```python
from build123d import *

# Parameters (mm, degrees)
PAD001_DEPTH      = 5
THICKNESS001_T    = 1.5
BOX_W             = 2
BOX_H             = 8
BOX_DEPTH         = 5
BOX001_W          = 2
BOX001_H          = 8
BOX001_DEPTH      = 5
BOX002_W          = 2
BOX002_H          = 6
BOX002_DEPTH      = 5
BOX003_W          = 2
BOX003_H          = 6
BOX003_DEPTH      = 5
CYLINDER001_W     = 3
CYLINDER001_H     = 5
CYLINDER001_ANGLE = 180
BOX005_W          = 6
BOX005_H          = 0.6
BOX005_DEPTH      = 5
CYLINDER005_W     = 3
CYLINDER005_H     = 5
CYLINDER005_ANGLE = 180
BOX007_W          = 6
BOX007_H          = 0.6
BOX007_DEPTH      = 5
SKETCH002_R       = 2.65
SKETCH002_R_2     = 1.25
SKETCH002_R_3     = 1
SKETCH002_W       = 5.3
SKETCH002_H       = 10.4
POCKET_DEPTH      = 6.501
BOX008_W          = 8
BOX008_H          = 2
BOX008_DEPTH      = 4.9
BOX009_W          = 8
BOX009_H          = 2
BOX009_DEPTH      = 4.9
SKETCH006_R       = 2.65
PAD003_DEPTH      = 3.5
SKETCH007_R       = 1.35
POCKET002_DEPTH   = 3.5


with BuildPart() as part:
    # Sketch001 → Pad001 (new body)
    with BuildSketch(Plane.XY):
        with BuildLine():
            Line((2, 31.1), (55.5, 31.1))
            ThreePointArc((57.6, 29), (56.984924, 30.484924), (55.5, 31.1))
            Line((57.6, 29), (57.6, 2))
            ThreePointArc((55.5, -0.1), (56.984924, 0.515076), (57.6, 2))
            Line((55.5, -0.1), (2, -0.1))
            ThreePointArc((-0.1, 2), (0.515076, 0.515076), (2, -0.1))
            Line((-0.1, 2), (-0.1, 29))
            ThreePointArc((2, 31.1), (0.515076, 30.484924), (-0.1, 29))
        make_face()
    extrude(amount=PAD001_DEPTH)

    # Thickness001
    thickness001_openings = [part.faces().sort_by_distance(p)[0] for p in [
        (28.75, 15.5, 0),
    ]]
    offset(amount=THICKNESS001_T, openings=thickness001_openings)

    # Box → Box (cut)
    with BuildSketch(Plane(origin=(57.5, 1.5, 0), x_dir=(1, 0, 0), z_dir=(0, 0, 1))):
        with Locations((1, 4)):
            Rectangle(BOX_W, BOX_H)
    extrude(amount=BOX_DEPTH, mode=Mode.SUBTRACT)

    # Box001 → Box001 (cut)
    with BuildSketch(Plane(origin=(57.5, 11.08, 0), x_dir=(1, 0, 0), z_dir=(0, 0, 1))):
        with Locations((1, 4)):
            Rectangle(BOX001_W, BOX001_H)
    extrude(amount=BOX001_DEPTH, mode=Mode.SUBTRACT)

    # Box002 → Box002 (cut)
    with BuildSketch(Plane(origin=(57.5, 20.575, 0), x_dir=(1, 0, 0), z_dir=(0, 0, 1))):
        with Locations((1, 3)):
            Rectangle(BOX002_W, BOX002_H)
    extrude(amount=BOX002_DEPTH, mode=Mode.SUBTRACT)

    # Box003 → Box003 (cut)
    with BuildSketch(Plane(origin=(-2, 10.35, 0), x_dir=(1, 0, 0), z_dir=(0, 0, 1))):
        with Locations((1, 3)):
            Rectangle(BOX003_W, BOX003_H)
    extrude(amount=BOX003_DEPTH, mode=Mode.SUBTRACT)

    # Cylinder001 → Cylinder001 (revolve)
    with BuildSketch(Plane(origin=(16, 0.5, 0), x_dir=(1, 0, 0), z_dir=(0, -1, 0))):
        with Locations((1.5, 2.5)):
            Rectangle(CYLINDER001_W, CYLINDER001_H)
    revolve(axis=Axis((16, 0.5, 0), (0, 0, 1)), revolution_arc=CYLINDER001_ANGLE)

    # Box005 → Box005 (join)
    with BuildSketch(Plane(origin=(13, -0.1, 0), x_dir=(1, 0, 0), z_dir=(0, 0, 1))):
        with Locations((3, 0.3)):
            Rectangle(BOX005_W, BOX005_H)
    extrude(amount=BOX005_DEPTH)

    # Cylinder005 → Cylinder005 (revolve)
    with BuildSketch(Plane(origin=(42.25, 30.5, 0), x_dir=(-1, 0, 0), z_dir=(0, 1, 0))):
        with Locations((1.5, 2.5)):
            Rectangle(CYLINDER005_W, CYLINDER005_H)
    revolve(axis=Axis((42.25, 30.5, 0), (0, 0, 1)), revolution_arc=CYLINDER005_ANGLE)

    # Box007 → Box007 (join)
    with BuildSketch(Plane(origin=(39.25, 30.5, 0), x_dir=(1, 0, 0), z_dir=(0, 0, 1))):
        with Locations((3, 0.3)):
            Rectangle(BOX007_W, BOX007_H)
    extrude(amount=BOX007_DEPTH)

    # Sketch002 → Pocket (cut, through all)
    with BuildSketch(Plane.XY):
        with Locations((47.135, 17.52)):
            Circle(SKETCH002_R)
        with Locations((16, 0.5)):
            Circle(SKETCH002_R_2)
        with Locations((42.25, 30.5)):
            Circle(SKETCH002_R_2)
        with Locations((45.15, 2.85)):
            Circle(SKETCH002_R_3)
        with Locations((33.1, 27.275)):
            Circle(SKETCH002_R_3)
        with Locations((3.6, 25.39)):
            Rectangle(SKETCH002_W, SKETCH002_H)
        with Locations((47.2, 25.7)):
            Rectangle(SKETCH002_W, SKETCH002_H)
        with BuildLine():
            Line((30.2, 2.925), (37, 2.925))
            ThreePointArc((37, 2.925), (37.919239, 3.305761), (38.3, 4.225))
            Line((38.3, 5.125), (38.3, 4.225))
            ThreePointArc((38.3, 5.125), (37.919239, 6.044239), (37, 6.425))
            Line((37, 6.425), (30.2, 6.425))
            ThreePointArc((30.2, 6.425), (29.280761, 6.044239), (28.9, 5.125))
            Line((28.9, 5.125), (28.9, 4.225))
            ThreePointArc((28.9, 4.225), (29.280761, 3.305761), (30.2, 2.925))
        make_face()
    extrude(amount=POCKET_DEPTH, mode=Mode.SUBTRACT)

    # Cone → Cone (revolve, cut)
    with BuildSketch(Plane(origin=(16, 0.5, 5.8), x_dir=(1, 0, 0), z_dir=(0, -1, 0))):
        Polygon((0, 0), (1.15, 0), (1.75, 0.7), (0, 0.7), align=None)
    revolve(axis=Axis((16, 0.5, 5.8), (0, 0, 1)), mode=Mode.SUBTRACT)

    # Cone001 → Cone001 (revolve, cut)
    with BuildSketch(Plane(origin=(42.25, 30.5, 5.8), x_dir=(1, 0, 0), z_dir=(0, -1, 0))):
        Polygon((0, 0), (1.15, 0), (1.75, 0.7), (0, 0.7), align=None)
    revolve(axis=Axis((42.25, 30.5, 5.8), (0, 0, 1)), mode=Mode.SUBTRACT)

    # Box008 → Box008 (cut)
    with BuildSketch(Plane(origin=(10.35, 31, 0), x_dir=(1, 0, 0), z_dir=(0, 0, 1))):
        with Locations((4, 1)):
            Rectangle(BOX008_W, BOX008_H)
    extrude(amount=BOX008_DEPTH, mode=Mode.SUBTRACT)

    # Box009 → Box009 (cut)
    with BuildSketch(Plane(origin=(21.82, 31, 0), x_dir=(1, 0, 0), z_dir=(0, 0, 1))):
        with Locations((4, 1)):
            Rectangle(BOX009_W, BOX009_H)
    extrude(amount=BOX009_DEPTH, mode=Mode.SUBTRACT)

    # Sketch006 → Pad003 (join)
    with BuildSketch(Plane.XY.offset(5)):
        with Locations((14.8, 22.4)):
            Circle(SKETCH006_R)
        with Locations((49.8, 5.4)):
            Circle(SKETCH006_R)
        with Locations((40.8, 22.4)):
            Circle(SKETCH006_R)
        with Locations((14.8, 5.4)):
            Circle(SKETCH006_R)
    extrude(amount=-PAD003_DEPTH)

    # Sketch007 → Pocket002 (cut)
    with BuildSketch(Plane.XY.offset(6.5)):
        with Locations((14.8, 22.4)):
            Circle(SKETCH007_R)
        with Locations((49.8, 5.4)):
            Circle(SKETCH007_R)
        with Locations((40.8, 22.4)):
            Circle(SKETCH007_R)
        with Locations((14.8, 5.4)):
            Circle(SKETCH007_R)
    extrude(amount=-POCKET002_DEPTH, mode=Mode.SUBTRACT)


solid = part.part
```
For this review, take the finished solid that the model builds, in its own axes (mm). A direction names the side the tool comes from. Round coordinates to 2 decimals unless told otherwise and drop trailing zeros. Write each loop counter-clockwise with the first axis right and the second up, starting at its lowest first coordinate (ties: lowest second). Pieces come first, ordered by that corner, then holes. Notation, with made-up numbers: (86, 62) -> (101, 62) arc R34 cw to (101, 100) -> close; hole circle Ø10 at (63.5, 63). An arc over 180 degrees is marked (long way). One line per question, with ' | ' between items. Start each with the question number.
(1) Add section B-B, the plane x = 33. Write out the cut boundary in (y, z) (3 decimals).
(2) Add section C-C, the plane x = 9. Write out the cut boundary in (y, z), plus the area to 3 significant figures.
(3) Add section A-A, the plane y = 17.52. Write out the cut boundary in (x, z) (3 decimals), plus the area to 3 significant figures.
(4) For line 1 along Y through (x, z) = (16, 3.55); line 2 along Y through (x, z) = (48, 2); line 3 along Y through (x, z) = (45.5, 3.25), list the stretches that pass through material, from the lowest coordinate up. Write a range as from..to.
(5) Insertion check: P1, Ø0.8, axis at x = 58, z = 3, coming from the +Y side; P2, Ø6, axis at x = 47.135, y = 17.52, coming from the -Z side; P3, Ø1.2, axis at y = 32, z = 3, coming from the +X side. Each pin has a flat end and moves straight along its axis. Give the tip position at first contact, or say it passes through.
(6) Add section D-D, the plane z = 4.25. Give the number of separate pieces and of enclosed holes in the cut face, plus the area to 3 significant figures.
(7) Tool access review of faces 1 (the face through (-1, 16.35, 2)), 2 (the face through (39.45, 22.46, 4.77)), 3 (the face through (37.929, 6.034, 5.74)): name each direction out of +Z, -Z, +X, -X, +Y, -Y from which nothing blocks a thin tool from reaching the whole face with its end or side.
(8) Mouldability with a two-part tool opening along Y and no side actions: class faces 4 (the face through (57, 30.47, 2.46)), 5 (the face through (17.088, 3.296, 2.535)), 6 (the face through (59.1, 10, 2)) as released by +Y, released by -Y, zero draft, split by the parting line, or undercut.
Answer list:
1) outline: (-1.6, 0) -> (-0.1, 0) -> (-0.1, 5) -> (2.925, 5) -> (2.925, 6.5) -> (-0.1, 6.5) arc R1.5 ccw to (-1.6, 5) -> close; (6.425, 5) -> (26.28, 5) -> (26.28, 6.5) -> (6.425, 6.5) -> close; (28.27, 5) -> (31.1, 5) -> (31.1, 0) -> (32.6, 0) -> (32.6, 5) arc R1.5 ccw to (31.1, 6.5) -> (28.27, 6.5) -> close
2) outline: (-1.6, 0) -> (-0.1, 0) -> (-0.1, 5) -> (31.1, 5) -> (31.1, 0) -> (32.6, 0) -> (32.6, 5) arc R1.5 ccw to (31.1, 6.5) -> (-0.1, 6.5) arc R1.5 ccw to (-1.6, 5) -> close | area: 65.3 mm²
3) outline: (-1.6, 0) -> (-0.1, 0) -> (-0.1, 5) -> (44.485, 5) -> (44.485, 6.5) -> (-0.1, 6.5) arc R1.5 ccw to (-1.6, 5) -> close; (49.785, 5) -> (59.1, 5) arc R1.5 ccw to (57.6, 6.5) -> (49.785, 6.5) -> close | area: 89.6 mm²
4) line 1: -1.6..-0.75, 1.75..4.78, 6.02..7.76, 20.04..21.78, 23.02..24.76 | line 2: -1.6..-0.1, 3.46..7.34, 31.1..32.6 | line 3: -1.6..-0.1, 31.1..32.6
5) P1: y = 31.92 | P2: z = 5 | P3: x = 58.18
6) separate pieces: 9 | enclosed holes: 6 | area: 291 mm²
7) face 1: -Z, +X, -X | face 2: +Z | face 3: +Z, -Z
8) face 4: undercut | face 5: undercut | face 6: zero draft
